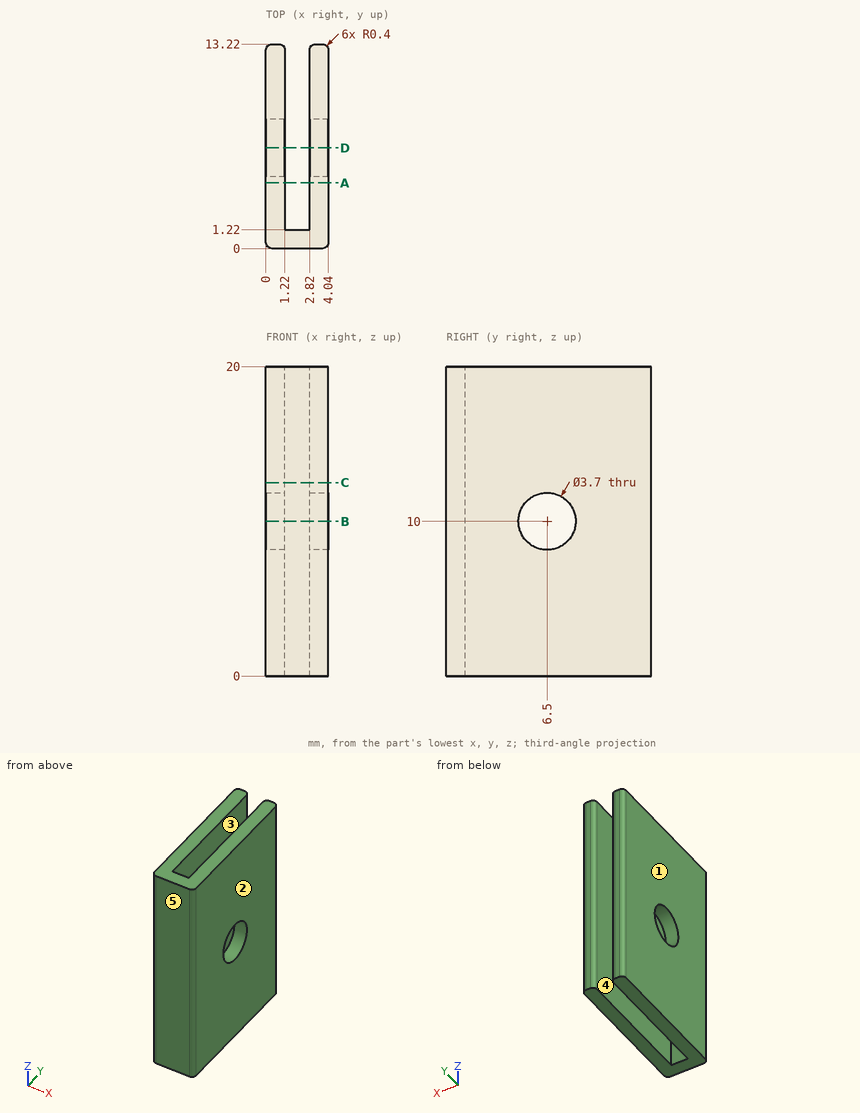
Could you check a few things on this drawing? It's one solid part, dimensions in mm from its lowest x, y, z. A direction names the side the tool comes from. Give positions to 0.01 mm unless a question says otherwise; leave off trailing zeros. Order: outer loops, then holes, each group sorted by start corner. A loop starts at its lowest first (then second) coordinate and runs counter-clockwise, first axis right, second up. Notation, with made-up numbers: (27.25, -26.5) -> (78.25, -26.5) arc R24 ccw to (78.25, 10.5) -> close; hole circle Ø5 at (13.25, 13). An arc over 180 degrees is marked (long way). Use CSV: the item, a comma, the result in double quotes. Start each with the question number.
Item 1: Thinking about a two-plate mould opening in X: for the marked faces 1, 2 and 3, which applies, pulls with the +X half, pulls with the -X half, needs draft (parallel to the pull), parting line crosses it, or undercut?
Item 2: If I drill on probe 1 along X at (y, z) = (11.5, 8.25); probe 2 along Y at (x, z) = (3.2, 10); probe 3 along Y at (x, z) = (2.5, 9), over which ranges is the centre line in solid material (lowest first)? Write a range as [from, to].
Item 3: On a 3-axis mill with a long thin cutter (end or side, diameter ignored), from which of +Z, -Z, +X, -X, +Y, -Y can I reach the whole of each face in a straight line? I mean the marked faces 4 and 5. Say none if no direction works.
Item 4: I'm going to push flat-ended pins straight in: P1, Ø3.5, axis at y = 7, z = 10, coming from the -X side; P2, Ø1.3, axis at x = 2.5, z = 10, coming from the +Y side. Where does each tip first touch, or does it pass through?
Item 5: Suppose I cut it at B-B (z = 10). List the corners of the cut face in (x, y) for me.
Item 6: Suppose I cut it at C-C (z = 12.5). List the corners of the cut face in (x, y) for me.
Item 7: Suppose I cut it at D-D (y = 6.5). List the corners of the cut face in (x, z) for me.
Item 8: Suppose I cut it at A-A (y = 4.25). List the corners of the cut face in (x, z) for me, and give its area (3 significant figures).
Answer block:
1,face 1,"pulls with the -X half"
1,face 2,"pulls with the +X half"
1,face 3,"undercut"
2,probe 1,"x = [0, 1.22], [2.82, 4.04]"
2,probe 2,"y = [0, 4.65], [8.35, 13.22]"
2,probe 3,"y = [0, 1.22]"
3,face 4,"+Z, -Z, +Y"
3,face 5,"+Z, -Z, +X, -X, -Y"
4,P1,"stops at x = 0"
4,P2,"stops at y = 13.21"
5,outline,"(0, 0.4) arc R0.4 ccw to (0.4, 0) -> (3.64, 0) arc R0.4 ccw to (4.04, 0.4) -> (4.04, 4.65) -> (2.82, 4.65) -> (2.82, 1.22) -> (1.22, 1.22) -> (1.22, 4.65) -> (0, 4.65) -> close; (0, 8.35) -> (1.22, 8.35) -> (1.22, 12.82) arc R0.4 ccw to (0.82, 13.22) -> (0.4, 13.22) arc R0.4 ccw to (0, 12.82) -> close; (2.82, 8.35) -> (4.04, 8.35) -> (4.04, 12.82) arc R0.4 ccw to (3.64, 13.22) -> (3.22, 13.22) arc R0.4 ccw to (2.82, 12.82) -> close"
6,outline,"(0, 0.4) arc R0.4 ccw to (0.4, 0) -> (3.64, 0) arc R0.4 ccw to (4.04, 0.4) -> (4.04, 12.82) arc R0.4 ccw to (3.64, 13.22) -> (3.22, 13.22) arc R0.4 ccw to (2.82, 12.82) -> (2.82, 1.22) -> (1.22, 1.22) -> (1.22, 12.82) arc R0.4 ccw to (0.82, 13.22) -> (0.4, 13.22) arc R0.4 ccw to (0, 12.82) -> close"
7,outline,"(0, 0) -> (1.22, 0) -> (1.22, 8.15) -> (0, 8.15) -> close; (0, 11.85) -> (1.22, 11.85) -> (1.22, 20) -> (0, 20) -> close; (2.82, 0) -> (4.04, 0) -> (4.04, 8.15) -> (2.82, 8.15) -> close; (2.82, 11.85) -> (4.04, 11.85) -> (4.04, 20) -> (2.82, 20) -> close"
8,outline,"(0, 0) -> (1.22, 0) -> (1.22, 20) -> (0, 20) -> close; (2.82, 0) -> (4.04, 0) -> (4.04, 20) -> (2.82, 20) -> close"
8,area,"48.8 mm^2"
